```python
from build123d import *

# Parameters (mm, degrees)
F0_R     = 2.032
F1_DEPTH = 6.35
F0_R_2   = 12.7
F2_DEPTH = 101.6


# Not quite as in the source:
# - a fillet or chamfer that OpenCascade refuses, or shapes differently, is made with other operations: its cross-section is extruded or revolved along the edge and cut away or added
# - the program builds the solid bodies; features that only make, move or delete a surface that nothing else refers to are left out


with BuildPart() as f1:
    # F0 (on Front) → F1 (new body)
    with BuildSketch(Plane.XZ):
        Polygon((-5.4516299168, -3.1475), (0, -6.295), (5.4516299168, -3.1475), (5.4516299168, 3.1475), (0, 6.295), (-5.4516299168, 3.1475), align=None)
        Circle(F0_R, mode=Mode.SUBTRACT)
    extrude(amount=F1_DEPTH)

    # F0 (on Front) → F2 (join)
    with BuildSketch(Plane.XZ):
        Circle(F0_R_2)
        Polygon((5.4516299168, -3.1475), (0, -6.295), (-5.4516299168, -3.1475), (-5.4516299168, 3.1475), (0, 6.295), (5.4516299168, 3.1475), align=None, mode=Mode.SUBTRACT)
    extrude(amount=F2_DEPTH)

    # F3: fillet of radius 7.62 on 1 edges, made by hand

    # F3_s1 → F3_t2 (revolve, cut)
    with BuildSketch(Plane.XY):
        with BuildLine():
            ThreePointArc((12.7, -93.98), (10.4681536726, -99.3681536726), (5.08, -101.6))
            Line((5.08, -101.6), (12.7, -101.6))
            Line((12.7, -101.6), (12.7, -93.98))
        make_face()
    revolve(axis=Axis((0, -101.6, 0), (0, -1, 0)), mode=Mode.SUBTRACT)


solid = f1.part
```
Check sheet for the modelled part. Datum: model origin and axes. Units: mm. A direction names the side the tool comes from. Give positions to 0.01 mm unless a question says otherwise; leave off trailing zeros. Order: outer loops, then holes, each group sorted by start corner. A loop starts at its lowest first (then second) coordinate and runs counter-clockwise, first axis right, second up. Notation, with made-up numbers: M 56,63.5 L 114,63.5 A9 cw 114,72.5 Z; hole C 73.25,88 d9. An arc over 180 degrees is marked long. Answer in a Markdown table with one row per item. Add a question column.
Q1. Sectioned sample at A-A, the plane y = -19. Record the boundary of the cut face in (x, z) (1 decimal).
Q2. Gauge pin test, flat ends, axial feed: pin 1 Ø6 at (x, y) = (9, -36) entering from +Z; pin 2 Ø2 at (y, z) = (-82.5, -7) entering from -X; pin 3 Ø2 at (x, z) = (8, -5.5) entering from -Y. Record the tip position at first contact, or that the pin passes through.
Q3. Access from +Z, -Z, +X, -X, +Y, -Y to the whole of each face (thin tool, end or side, straight path). Record for faces 1 (the cylindrical face through (-0.44, -3.131, -1.984)), 2 (the flat face through (2.76, -53.3, -4.7)).
Q4. Release check for a two-part mould opening along Z. For faces 3 (the flat face through (2.69, -53.3, 4.74)), 4 (the cylindrical face through (-2.75, -46.33, -12.4)), 5 (the flat face through (3, 0, 0)) record: released by +Z, released by -Z, zero draft, split by the parting line, or undercut.
Q5. Thickness scan on L1, parallel to Z at x = 0, y = -32.5 (3 decimals); L2, parallel to Y at x = -4, z = -2; L3, parallel to Z at x = 0, y = -2.25. Record the ranges inside material, lowest first.
Verdict:
| question | item | result |
|---|---|---|
| 1 | outline | C 0,0 d25.4; hole M -5.5,-3.1 L 0,-6.3 L 5.5,-3.1 L 5.5,3.1 L 0,6.3 L -5.5,3.1 Z |
| 2 | pin 1 | z = 11.19 |
| 2 | pin 2 | x = -11.19 |
| 2 | pin 3 | y = -100.68 |
| 3 | face 1 | +Y, -Y |
| 3 | face 2 | -Y |
| 4 | face 3 | undercut |
| 4 | face 4 | split by the parting line |
| 4 | face 5 | zero draft |
| 5 | L1 | -12.7 to -6.295, 6.295 to 12.7 |
| 5 | L2 | -6.35 to 0 |
| 5 | L3 | -12.7 to -2.03, 2.03 to 12.7 |
